Autodesk Fusion 360 part; units mm, degrees
sketch "Sketch1" plane through (0, 0, 0) normal (0, 1, 0) x (1, 0, 0)
  line L0 (0, 0) -> (50, 0)
  line L1 (50, 0) -> (50, 36.5)
  line L2 (50, 36.5) -> (0, 36.5)
  line L3 (0, 36.5) -> (0, 0)
  line L4 (0, 36.5) -> (50, 0)
  line L5 (50, 36.5) -> (0, 0)
  circle A0 centre (25, 18.25) radius 3.5
  dimension "d1" = 50
  dimension "d2" = 36.5
  dimension "d3" = 7
extrude "Extrude1" add sketch "Sketch1" along normal blind 1 contours L0 L4 L5 A0 | L3 L4 L5 A0 | L1 L4 L5 A0 | L2 L4 L5 A0
Build history of the part. All positions in model axes, mm. Coordinates: 2 decimals unless noted, no trailing zeros. Order: outer loops, then holes, each group sorted by start corner. A loop starts at its lowest first (then second) coordinate and runs counter-clockwise, first axis right, second up. Notation, with made-up numbers: M -16,-21 L 40,-21 A21 ccw 40,15 Z; hole C -36.5,33.5 d11. An arc over 180 degrees is marked long. One line per question, with ' | ' between items. Start each with the question number.
1. Cut at B-B (x = 25). Write the cut outline in (y, z), plus the area to 3 significant figures.
2. Mould opens along Z. For faces 1 (the face through (26.88, 0.49, -15.3)), 2 (the face through (0, 0.5, -18.5)), 3 (the face through (24.7, 0.5, 0)) say: +Z half, -Z half, draft (parallel to the pull), parting line (faces both ways), or undercut.
3. Flat gauge pin, fed straight in: P1, Ø11, axis at x = 25, z = -18.25, coming from the -Y side. Where does the tip first touch, or does it go through?
4. Cut at A-A (z = -18.25). Write the cut outline in (x, y).
5. Cut at C-C (y = 0.55). Write the cut outline in (x, z).
6. Wall check: line 1 along X through (y, z) = (0.6, -18.25); line 2 along Z through (x, y) = (25, 0.45); line 3 along X through (y, z) = (0.75, -20). Give the ranges that are in metal, low to high. Write a range as [from, to].
The answers:
1) outline: M 0,-36.5 L 1,-36.5 L 1,-21.75 L 0,-21.75 Z; M 0,-14.75 L 1,-14.75 L 1,0 L 0,0 Z | area: 29.5 mm2
2) face 1: undercut | face 2: draft | face 3: +Z half
3) P1: stops at y = 0
4) outline: M 0,0 L 21.5,0 L 21.5,1 L 0,1 Z; M 28.5,0 L 50,0 L 50,1 L 28.5,1 Z
5) outline: M 0,-36.5 L 50,-36.5 L 50,0 L 0,0 Z; hole C 25,-18.25 d7
6) line 1: x = [0, 21.5], [28.5, 50] | line 2: z = [-36.5, -21.75], [-14.75, 0] | line 3: x = [0, 21.97], [28.03, 50]
